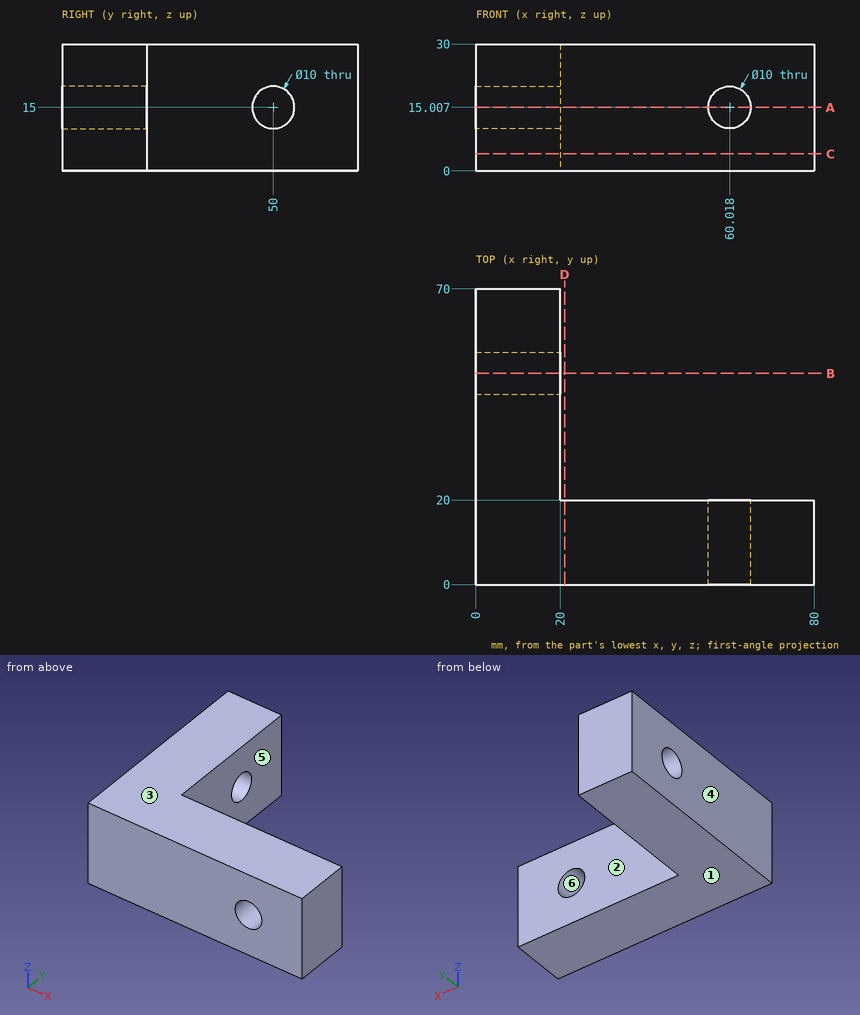
The drawing under review shows one solid part. Ordinate dimensions are in mm from its lowest x, y, z. A direction names the side the tool comes from. Coordinates: 2 decimals unless noted, no trailing zeros. Write each loop counter-clockwise with the first axis right and the second up, starting at its lowest first coordinate (ties: lowest second). Pieces come first, ordered by that corner, then holes. Notation, with made-up numbers: (10.5, 80) - (68.5, 80) arc R25 cw to (68.5, 114) - close; hole circle Ø7 at (-1, 29.25). An arc over 180 degrees is marked (long way). Answer as CSV lines item,"result".
(1) Mouldability with a two-part tool opening along X and no side actions: class the marked faces 3, 4, 5 and 6 as pulls with the +X half, pulls with the -X half, needs draft (parallel to the pull), parting line crosses it, or undercut.
Data:
face 3,"needs draft"
face 4,"pulls with the -X half"
face 5,"pulls with the +X half"
face 6,"undercut"
(2) We need section B-B (y = 50). Give the boundary of the cut face in (x, z).
Data:
outline,"(0, 0) - (20, 0) - (20, 10) - (0, 10) - close; (0, 20) - (20, 20) - (20, 30) - (0, 30) - close"
(3) We need section D-D (x = 21). Give the boundary of the cut face in (y, z), plus the area to 3 significant figures.
Data:
outline,"(0, 0) - (20, 0) - (20, 30) - (0, 30) - close"
area,"600 mm2"
(4) We need section A-A (z = 15). Give the boundary of the cut face in (x, y).
Data:
outline,"(0, 0) - (55.02, 0) - (55.02, 20) - (20, 20) - (20, 45) - (0, 45) - close; (0, 55) - (20, 55) - (20, 70) - (0, 70) - close; (65.02, 0) - (80, 0) - (80, 20) - (65.02, 20) - close"
(5) Tool access review of the marked faces 1 and 2: name each direction out of +Z, -Z, +X, -X, +Y, -Y from which nothing blocks a thin tool from reaching the whole face with its end or side.
Data:
face 1,"-Z, +X, -X, +Y, -Y"
face 2,"+Z, -Z, +X, +Y"
(6) For line 1 along Y through (x, z) = (11, 15); line 2 along Y through (x, z) = (53.5, 17.25), list the stretches that pass through material, from the lowest coordinate up. Write a range as [from, to].
Data:
line 1,"y = [0, 45], [55, 70]"
line 2,"y = [0, 20]"
(7) We need section C-C (z = 4). Give the boundary of the cut face in (x, y), plus the area to 3 significant figures.
Data:
outline,"(0, 0) - (80, 0) - (80, 20) - (20, 20) - (20, 70) - (0, 70) - close"
area,"2,600 mm2"
(8) Clearance check with flat-ended pins moving along their axes: pin 1 Ø1 at (y, z) = (41, 6.5) entering from +X; pin 2 Ø11.5 at (x, z) = (60.02, 15.01) entering from +Y. State where each tip first meets the part, or that it passes through.
Data:
pin 1,"stops at x = 20"
pin 2,"stops at y = 20"
